Could you check a few things on this model? Use its own coordinates, in mm. A direction names the side the tool comes from. Round coordinates to 2 decimals unless told otherwise and drop trailing zeros. Order: outer loops, then holes, each group sorted by start corner. A loop starts at its lowest first (then second) coordinate and runs counter-clockwise, first axis right, second up.
```python
from build123d import *

# Parameters (mm, degrees)
F0_R     = 75
F1_DEPTH = 90
F2_R     = 75
F2_W     = 420
F2_H     = 70
F3_DEPTH = 210
F4_SIZE  = 210


with BuildPart() as f1:
    # F0 (on Top) → F1 (new body)
    with BuildSketch(Plane.XY):
        with BuildLine():
            Line((-510, 0), (0, 0))
            Line((0, 0), (90, 90))
            Line((90, 90), (90, 210))
            Line((90, 210), (0, 300))
            Line((0, 300), (-330, 300))
            Line((-330, 300), (-510, 300))
            ThreePointArc((-510, 300), (-660, 150), (-510, 0))
        make_face()
        with Locations((-510, 150)):
            Circle(F0_R, mode=Mode.SUBTRACT)
    extrude(amount=F1_DEPTH)

    # F2 (on face) → F3 (join)
    with BuildSketch(Plane.XY.offset(90)):
        with BuildLine():
            Line((-330, 300), (-510, 300))
            ThreePointArc((-510, 300), (-660, 150), (-510, 0))
            Line((-510, 0), (-330, 0))
            Line((-330, 0), (-330, 115))
            Line((-330, 115), (-330, 185))
            Line((-330, 185), (-330, 300))
        make_face()
        with Locations((-510, 150)):
            Circle(F2_R, mode=Mode.SUBTRACT)
        with Locations((-120, 150)):
            Rectangle(F2_W, F2_H)
    extrude(amount=F3_DEPTH)

    # F4
    f4_edges = [f1.edges().sort_by_distance(p)[0] for p in [
        (90, 150, 300),
    ]]
    chamfer(f4_edges, length=F4_SIZE)


solid = f1.part
```
Q1. Imagine slicing it at D-D, the plane z = 191.5. Please give me the cut outline in (x, y).
Q2. I need wall thicknesses on L1, parallel to Y at x = -510, z = 178; L2, parallel to Z at x = -227, y = 261; L3, parallel to Y at x = -18, z = 173. Which ranges of each line are inside material? Lowest first, please.
Q3. Imagine slicing it at B-B, the plane z = 280. Please give me the cut outline in (x, y).
Q4. Imagine slicing it at C-C, the plane x = -131. Please give me the cut outline in (y, z), then the cut area to 3 significant figures.
Q5. Imagine slicing it at A-A, the plane y = 150. Please give me the cut outline in (x, z).
Q6. We'd pull the mould along X, two halves only. Please class faces 1 (the flat face through (-290, 152, 0)), 2 (the cylindrical face through (-659.964, 153.298, 147.9)), 3 (the cylindrical face through (-438.463, 172.528, 147.9)), 4 (the flat face through (44, 44, 44)): released by +X, released by -X, zero draft, split by the parting line, or undercut.
Q7. For P1, Ø3, axis at x = -556.5, z = 202, coming from the +Y side; P2, Ø12, axis at x = -256.5, z = 164, coming from the -Y side; P3, Ø4, axis at x = -180.5, y = 196.5, coming from the +Z side, each with a flat end and sliding along its axis, tell me the tip position at first contact or that it passes through.
Q8. For faces 5 (the flat face through (-394, 152, 300)), 6 (the flat face through (-170, 185, 194)), 7 (the flat face through (-123, 58, 90)), which set-ups out of +Z, -Z, +X, -X, +Y, -Y let a thin tool reach every point of the face, with its end or its side?
Filled in:
1. outline: (-510, 0) - (-330, 0) - (-330, 115) - (-11.5, 115) - (-11.5, 185) - (-330, 185) - (-330, 300) - (-510, 300) arc R150 ccw to start; hole circle Ø150 at (-510, 150)
2. L1: y = 0 to 75, 225 to 300
2. L2: z = 0 to 90
2. L3: y = 115 to 185
3. outline: (-510, 0) - (-330, 0) - (-330, 115) - (-100, 115) - (-100, 185) - (-330, 185) - (-330, 300) - (-510, 300) arc R150 ccw to start; hole circle Ø150 at (-510, 150)
4. outline: (0, 0) - (300, 0) - (300, 90) - (185, 90) - (185, 300) - (115, 300) - (115, 90) - (0, 90) - close
4. area: 41,700 mm2
5. outline: (-660, 0) - (-585, 0) - (-585, 300) - (-660, 300) - close; (-435, 0) - (90, 0) - (90, 90) - (-120, 300) - (-435, 300) - close
6. face 1: zero draft
6. face 2: released by -X
6. face 3: undercut
6. face 4: released by +X
7. P1: stops at y = 293.09
7. P2: stops at y = 115
7. P3: stops at z = 90
8. face 5: +Z, +X, -X, +Y, -Y
8. face 6: +Z, +X, +Y
8. face 7: +Z, +X, -Y
